Input: part model. Units: mm. Frame: model coordinates. A direction names the side the tool comes from. Round coordinates to 2 decimals unless told otherwise and drop trailing zeros. Order: outer loops, then holes, each group sorted by start corner. A loop starts at its lowest first (then second) coordinate and runs counter-clockwise, first axis right, second up. Notation, with made-up numbers: (27, -17.5) -> (65, -17.5) arc R19 cw to (65, 5.5) -> close; hole circle Ø2 at (-1, -14). An arc over 180 degrees is marked (long way). Use a Markdown table: item, result.
Autodesk Inventor part; units mm, degrees
ref_plane "Płaszczyzna konstrukcyjna1" through (1.875, 0, 0) normal (1, 0, 0) x (0, 1, 0)
ref_plane "Płaszczyzna konstrukcyjna2" through (-1.875, 0, 0) normal (1, 0, 0) x (0, 1, 0)
ref_plane "XZ Plane" through (0, 0, 0) normal (0, 1, 0) x (-1, 0, 0)
sketch "Szkic1" plane through (0, 0, 0) normal (0, 1, 0) x (-1, 0, 0)
  circle A0 centre (0, 0) radius 6.875
  circle A1 centre (0, 0) radius 4
  dimension "d0" = 13.75
  dimension "d1" = 8
extrude "Wyciągnięcie proste1" add sketch "Szkic1" along normal blind 4
sketch "Szkic2" plane through (0, 4, 0) normal (0, 1, 0) x (1, 0, 0)
  circle A0 centre (0, 0) radius 5.15
  circle A1 centre (0, 0) radius 4
  dimension "d4" = 10.3
extrude "Wyciągnięcie proste2" add sketch "Szkic2" along normal blind 11
ref_plane "Płaszczyzna konstrukcyjna1" through (1.875, 0, 0) normal (1, 0, 0) x (0, 1, 0)
sketch "Szkic3" plane through (1.875, 0, 0) normal (1, 0, 0) x (0, 1, 0)
  line L0 (15, 4) -> (15, -4)
  line L1 (0, -4) -> (0, 4)
  line L2 (4, 5.15) -> (15, 5.15)
  line L3 (4, -5.15) -> (15, -5.15)
  line L4 (15, -5.15) -> (15, 5.15)
  line L5 (15, 5.15) -> (11, 5.15)
  line L6 (11, 5.15) -> (11, -5.15)
  line L7 (11, -5.15) -> (15, -5.15)
  line L8 (15, -5.15) -> (15, 5.15)
  point P0 (0, 0)
  dimension "d8" = 4
extrude "Wyciągnięcie proste3" cut sketch "Szkic3" along normal through all
ref_plane "Płaszczyzna konstrukcyjna2" through (-1.875, 0, 0) normal (1, 0, 0) x (0, 1, 0)
sketch "Szkic4" plane through (-1.875, 0, 0) normal (1, 0, 0) x (0, 1, 0)
  line L0 (4, 5.15) -> (4, -5.15)
  line L1 (15, -4.7965) -> (11, -4.7965)
  line L2 (11, -4.7965) -> (11, 4.7965)
  line L3 (11, 4.7965) -> (15, 4.7965)
  line L4 (15, -4.7965) -> (15, 4.7965)
  line L5 (4, 5.15) -> (15, 5.15)
  line L6 (15, -6.2367) -> (11, -6.2367)
  line L7 (11, -6.2367) -> (11, 6.0914)
  line L8 (11, 6.0914) -> (15, 6.0914)
  line L9 (15, 6.0914) -> (15, -6.2367)
  point P0 (0, 0)
extrude "Wyciągnięcie proste4" cut sketch "Szkic4" against normal through all
properties part number "napinacz nakretki tr8"
1) Set-up query: faces 1 (the flat face through (-1.875, 13, 4)), 2 (the flat face through (1.875, 13, 4)), 3 (the flat face through (0, 15, -4.4)), 4 (the flat face through (-3, 4, 5)). Return all of +Z, -Z, +X, -X, +Y, -Y with unobstructed straight access to the full face (end or side cutting, diameter ignored); none if empty.
Results found:
| item | result |
|---|---|
| face 1 | +Z, -Z, -X, +Y |
| face 2 | +Z, -Z, +X, +Y |
| face 3 | +Z, -Z, +X, -X, +Y |
| face 4 | +Y |
2) Line query: L1, parallel to Z at x = 0, y = 6.75; L2, parallel to Y at x = 3.75, z = -3.25. Output: solid intervals per line, ascending. Write a range as [from, to].
Results found:
| item | result |
|---|---|
| L1 | z = [-5.15, -4], [4, 5.15] |
| L2 | y = [0, 11] |
3) Cut plane A-A on y = 7. Return loops of the section in (x, z), and give its area (3 significant figures).
Results found:
| item | result |
|---|---|
| outline | circle Ø10.3 at (0, 0); hole circle Ø8 at (0, 0) |
| area | 33.1 mm² |
4) Cut plane D-D on z = -1.25. Return loops of the section in (x, y).
Results found:
| item | result |
|---|---|
| outline | (-6.76, 0) -> (-3.8, 0) -> (-3.8, 11) -> (-5, 11) -> (-5, 4) -> (-6.76, 4) -> close; (3.8, 0) -> (6.76, 0) -> (6.76, 4) -> (5, 4) -> (5, 11) -> (3.8, 11) -> close |
5) Pin query (flat end, axial travel): pin 1 Ø5 at (y, z) = (12.5, 1.5) entering from +X; pin 2 Ø6 at (x, y) = (1.5, 12) entering from +Z; pin 3 Ø1 at (y, z) = (12.5, -4) entering from -X (3 decimals); pin 4 Ø5 at (x, z) = (0, 0) entering from -Y. Return the tip coordinate at first contact, or that it passes through.
Results found:
| item | result |
|---|---|
| pin 1 | stops at x = 5.15 |
| pin 2 | stops at z = 5.15 |
| pin 3 | stops at x = -1.875 |
| pin 4 | passes through |
6) Pull-direction query (Y, two-part tool) for faces 5 (the flat face through (-3, 0, -3)), 6 (the cylindrical face through (1.49, 1.97, 6.71)), 7 (the flat face through (4.2, 11, 0.1)); classes: +Y half, -Y half, draft (parallel to the pull), parting line (faces both ways), or undercut.
Results found:
| item | result |
|---|---|
| face 5 | -Y half |
| face 6 | draft |
| face 7 | +Y half |
7) Cut plane B-B on z = -3. Return loops of the section in (x, y).
Results found:
| item | result |
|---|---|
| outline | (-6.19, 0) -> (-2.65, 0) -> (-2.65, 11) -> (-4.19, 11) -> (-4.19, 4) -> (-6.19, 4) -> close; (2.65, 0) -> (6.19, 0) -> (6.19, 4) -> (4.19, 4) -> (4.19, 11) -> (2.65, 11) -> close |
